Source: three-view drawing plus pictorial views. Frame: mm from the lowest corner of the part. A direction names the side the tool comes from. Give positions to 0.01 mm unless a question says otherwise; leave off trailing zeros. Loops run counter-clockwise (first coordinate to the right, second up) from the corner with the lowest first, then second, coordinate; pieces in that order, holes last. Notation, with made-up numbers: (23, 67) - (64, 67) arc R28 ccw to (64, 101) - close; hole circle Ø11 at (-30.75, 69). An arc over 180 degrees is marked (long way). Answer as a JSON object with one key per item and string values.
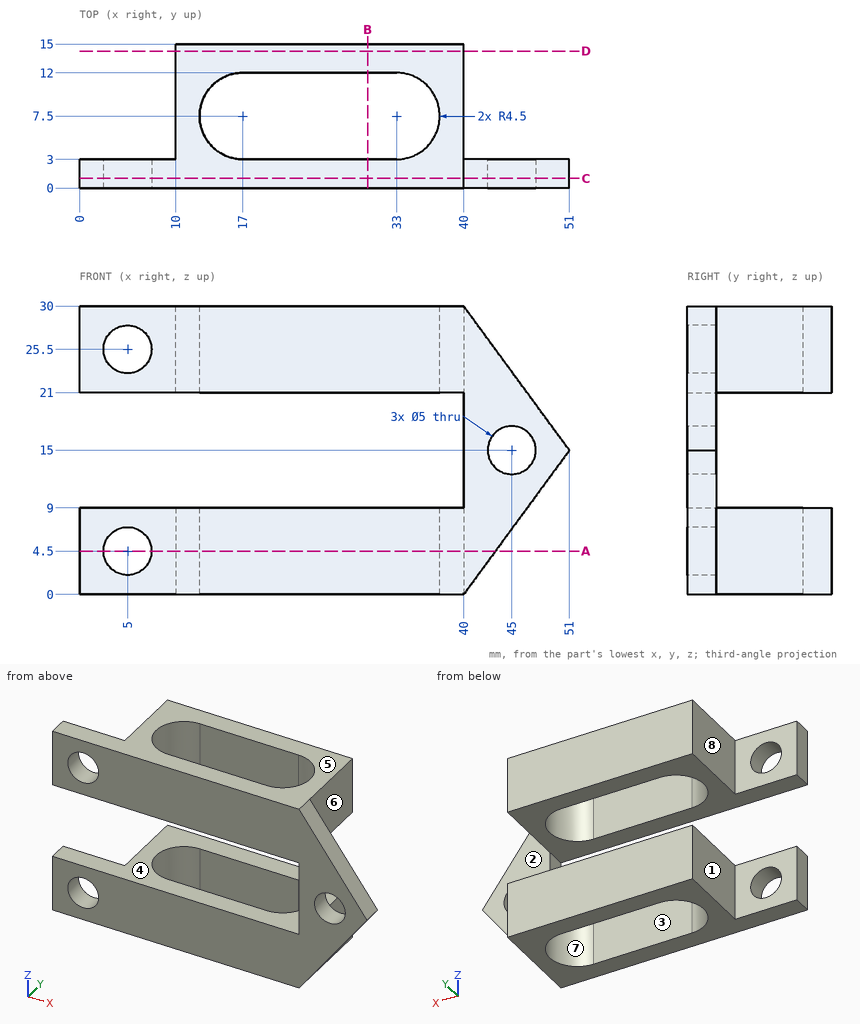
Item 1: Cut plane D-D (y = 14.25). Return loops of the section in (x, z), then the cut area to 3 significant figures.
Geometry check:
{"outline": "(10, 0) - (40, 0) - (40, 9) - (10, 9) - close; (10, 21) - (40, 21) - (40, 30) - (10, 30) - close", "area": "540 mm2"}
Item 2: Mould query, pull axis X, two halves, no side actions, for the marked faces 5, 6, 7 and 8. Classes: released by +X, released by -X, zero draft, split by the parting line, or undercut.
Geometry check:
{"face 5": "zero draft", "face 6": "released by +X", "face 7": "undercut", "face 8": "released by -X"}
Item 3: Access query for the marked faces 1, 2, 3 and 4. Directions: +Z, -Z, +X, -X, +Y, -Y. A direction counts if a zero-diameter tool reaches every point of the face in a straight line with its end or side. Return the directions, or none.
Geometry check:
{"face 1": "+Z, -Z, -X, +Y", "face 2": "+Z, -Z, +X, +Y", "face 3": "+Z, -Z", "face 4": "-X, +Y, -Y"}
Item 4: Contact query for flat-ended pins moving along their axis: P1, Ø5.5, axis at x = 44, z = 16.5, coming from the +Y side; P2, Ø1, axis at y = 4, z = 8.5, coming from the -X side; P3, Ø1.5, axis at y = 2, z = 13, coming from the -X side. Output: stop coordinate, or through.
Geometry check:
{"P1": "stops at y = 3", "P2": "stops at x = 10", "P3": "stops at x = 40"}
Item 5: Cut plane B-B (x = 30). Return loops of the section in (y, z), then the cut area to 3 significant figures.
Geometry check:
{"outline": "(0, 0) - (3, 0) - (3, 9) - (0, 9) - close; (0, 21) - (3, 21) - (3, 30) - (0, 30) - close; (12, 0) - (15, 0) - (15, 9) - (12, 9) - close; (12, 21) - (15, 21) - (15, 30) - (12, 30) - close", "area": "108 mm2"}
Item 6: Cut plane A-A (z = 4.5). Return loops of the section in (x, y), then the cut area to 3 significant figures.
Geometry check:
{"outline": "(0, 0) - (2.5, 0) - (2.5, 3) - (0, 3) - close; (7.5, 0) - (43.3, 0) - (43.3, 3) - (40, 3) - (40, 15) - (10, 15) - (10, 3) - (7.5, 3) - close; hole (17, 3) - (33, 3) arc R4.5 ccw to (33, 12) - (17, 12) arc R4.5 ccw to start", "area": "267 mm2"}
Item 7: Cut plane C-C (y = 1). Return loops of the section in (x, z), then the cut area to 3 significant figures.
Geometry check:
{"outline": "(0, 0) - (40, 0) - (51, 15) - (40, 30) - (0, 30) - (0, 21) - (40, 21) - (40, 9) - (0, 9) - close; hole circle Ø5 at (5, 4.5); hole circle Ø5 at (5, 25.5); hole circle Ø5 at (45, 15)", "area": "826 mm2"}
Item 8: Material intervals for line 1 (Z direction, x = 5, y = 1.55); line 2 (Y direction, x = 33, z = 21.25); line 3 (X direction, y = 0.8, z = 15), sorted ascending. Write a range as [from, to].
Geometry check:
{"line 1": "z = [0, 2], [7, 9], [21, 23], [28, 30]", "line 2": "y = [0, 3], [12, 15]", "line 3": "x = [40, 42.5], [47.5, 51]"}
